Print and shaded views of the part. All mm, measured from the part's lowest x, y and z. A direction names the side the tool comes from. Round coordinates to 2 decimals unless told otherwise and drop trailing zeros. Loops run counter-clockwise (first coordinate to the right, second up) from the corner with the lowest first, then second, coordinate; pieces in that order, holes last. Notation, with made-up numbers: (-27.5, 56.5) - (27.5, 56.5) arc R27 cw to (27.5, 72.5) - close; hole circle Ø2 at (18.5, 33.5). An arc over 180 degrees is marked (long way). Use one line per item in the form item = value. Start each with the question number.
Q1. 3-axis set-ups, long thin cutter, end or side, ignore diameter. For the marked faces 5 and 6: which of +Z, -Z, +X, -X, +Y, -Y reach the whole face in a straight line?
Q2. Pin check, flat tips, straight feed: pin 1 (2.5 mm diameter, centred on y = 6, z = 2.5, fed in from +X); pin 2 (1.6 mm diameter, centred on x = 7.62, z = 2.54, fed in from -Y); pin 3 (3 mm diameter, centred on x = 7, z = 2, fed in from +Y). Stop position of each tip, or through.
Q3. Mould opens along X. For the marked faces 1, 2, 3 and 4 say: released by +X, released by -X, zero draft, split by the parting line, or undercut.
Q4. Drill centre lines: line 1 (Z direction, x = 7.62, y = 0.95); line 2 (Y direction, x = 0.8, z = 2.54); line 3 (Y direction, x = 8.75, z = 0.6). Where is each one in solid material? Low to high.
Q5. Saw through at D-D (y = 1.5). Give the cut face in (x, z).
Q6. Saw through at A-A (y = 6.35). Give the cut face in (x, z), then the cut area to 3 significant figures.
Q7. Saw through at B-B (z = 2.54). Give the cut face in (x, y).
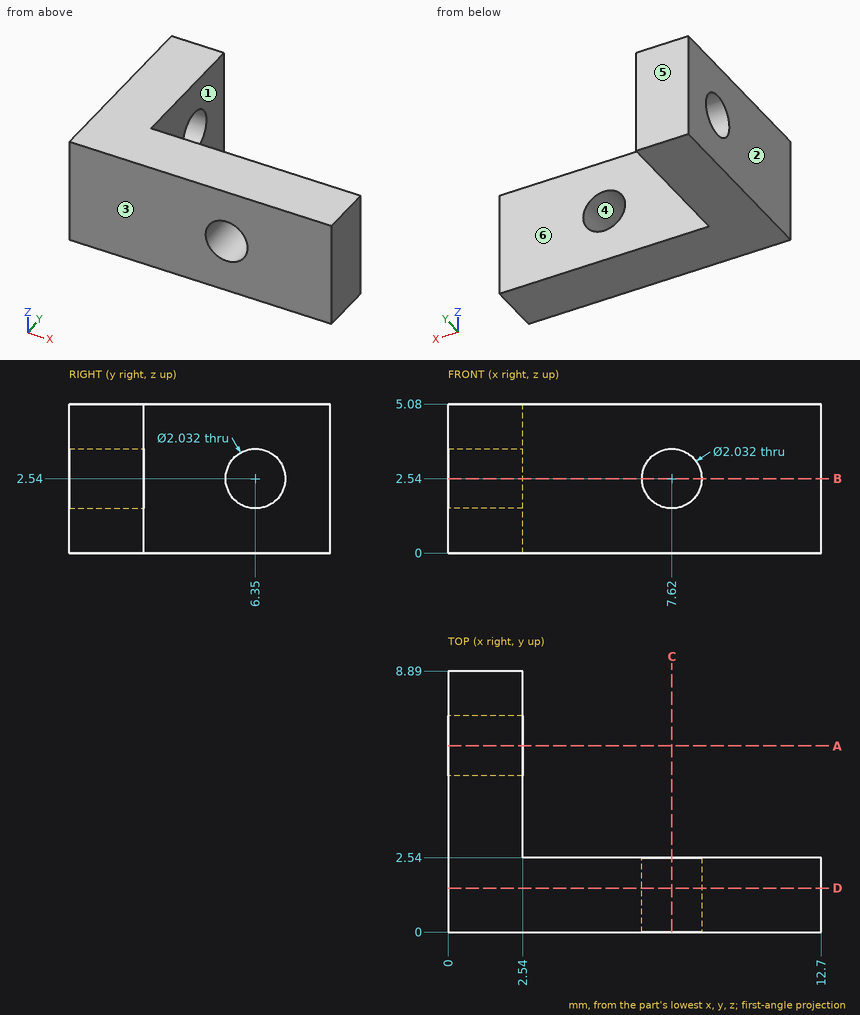
Report:
q1.face_5 = +Z, -Z, +X, -X, +Y
q1.face_6 = +Z, -Z, +X, +Y
q2.pin_1 = 2.54
q2.pin_2 = through
q2.pin_3 = 2.54
q3.face_1 = released by +X
q3.face_2 = released by -X
q3.face_3 = zero draft
q3.face_4 = undercut
q4.line_1 = 0 to 1.52, 3.56 to 5.08
q4.line_2 = 0 to 5.33, 7.37 to 8.89
q4.line_3 = 0 to 2.54
q5.outline = (0, 0) - (12.7, 0) - (12.7, 5.08) - (0, 5.08) - close; hole circle Ø2.03 at (7.62, 2.54)
q6.outline = (0, 0) - (2.54, 0) - (2.54, 1.52) - (0, 1.52) - close; (0, 3.56) - (2.54, 3.56) - (2.54, 5.08) - (0, 5.08) - close
q6.area = 7.74 mm²
q7.outline = (0, 0) - (6.6, 0) - (6.6, 2.54) - (2.54, 2.54) - (2.54, 5.33) - (0, 5.33) - close; (0, 7.37) - (2.54, 7.37) - (2.54, 8.89) - (0, 8.89) - close; (8.64, 0) - (12.7, 0) - (12.7, 2.54) - (8.64, 2.54) - close
